Geometry check sheet. Reference: drawing and pictorial views, mm from the part's lowest x, y, z. Coordinates: 2 decimals unless noted, no trailing zeros. Loops run counter-clockwise (first coordinate to the right, second up) from the corner with the lowest first, then second, coordinate; pieces in that order, holes last. Notation, with made-up numbers: (33.25, 68.5) - (88.25, 68.5) arc R17 cw to (88.25, 96.5) - close; hole circle Ø1 at (79, 46). An arc over 180 degrees is marked (long way). One line per item, written item: value.
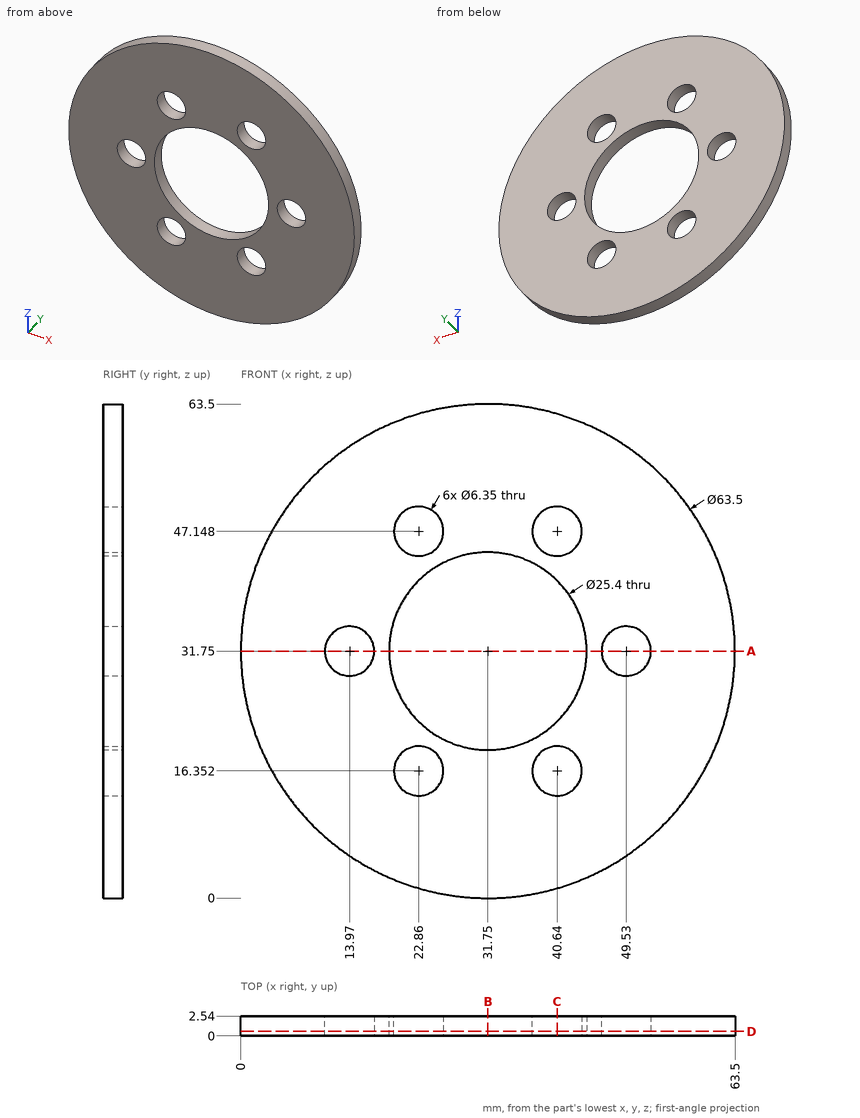
(1) Cross-section at A-A on z = 31.75. Record the cut outline in (x, y) (3 decimals).
Reply:
outline: (0, 0) - (10.795, 0) - (10.795, 2.54) - (0, 2.54) - close; (17.145, 0) - (19.05, 0) - (19.05, 2.54) - (17.145, 2.54) - close; (44.45, 0) - (46.355, 0) - (46.355, 2.54) - (44.45, 2.54) - close; (52.705, 0) - (63.5, 0) - (63.5, 2.54) - (52.705, 2.54) - close
(2) Cross-section at D-D on y = 0.6. Record the cut outline in (x, z) (3 decimals), and give its area (3 significant figures).
Reply:
outline: circle Ø63.5 at (31.75, 31.75); hole circle Ø6.35 at (13.97, 31.75); hole circle Ø25.4 at (31.75, 31.75); hole circle Ø6.35 at (22.86, 16.352); hole circle Ø6.35 at (22.86, 47.148); hole circle Ø6.35 at (40.64, 16.352); hole circle Ø6.35 at (40.64, 47.148); hole circle Ø6.35 at (49.53, 31.75)
area: 2,470 mm2
(3) Cross-section at B-B on x = 31.75. Record the cut outline in (y, z), and give its area (3 significant figures).
Reply:
outline: (0, 0) - (2.54, 0) - (2.54, 19.05) - (0, 19.05) - close; (0, 44.45) - (2.54, 44.45) - (2.54, 63.5) - (0, 63.5) - close
area: 96.8 mm2
(4) Cross-section at C-C on x = 40.64. Record the cut outline in (y, z), and give its area (3 significant figures).
Reply:
outline: (0, 1.27) - (2.54, 1.27) - (2.54, 13.18) - (0, 13.18) - close; (0, 19.53) - (2.54, 19.53) - (2.54, 22.68) - (0, 22.68) - close; (0, 40.82) - (2.54, 40.82) - (2.54, 43.97) - (0, 43.97) - close; (0, 50.32) - (2.54, 50.32) - (2.54, 62.23) - (0, 62.23) - close
area: 76.5 mm2
(5) Material ranges on probe 1 along X at (y, z) = (2.2, 15.5); probe 2 along Z at (x, y) = (40.64, 0.6); probe 3 along X at (y, z) = (2.15, 30), recorded low to high. Write a range as from..to.
Reply:
probe 1: 4.47..19.8, 25.92..37.58, 43.7..59.03
probe 2: 1.27..13.18, 19.53..22.68, 40.82..43.97, 50.32..62.23
probe 3: 0.05..11.32, 16.62..19.17, 44.33..46.88, 52.18..63.45
